Could you check a few things on this model? Use its own coordinates, in mm. A direction names the side the tool comes from. Coordinates: 2 decimals unless noted, no trailing zeros. Order: outer loops, then holes, each group sorted by start corner. A loop starts at its lowest first (then second) coordinate and runs counter-clockwise, first axis right, second up.
```python
from build123d import *

# Parameters (mm, degrees)
SKETCH1_R                  = 25.4
BOSS_EXTRUDE1_DEPTH        = 25.4
CUT_EXTRUDE1_START         = -12.7
SKETCH2_R                  = 25.4
SKETCH2_R_2                = 15.875
CUT_EXTRUDE1_DEPTH         = 12.7
F_3_4_0_7500_DOWEL_HOLE1_D = 19.05
F_3_0MM_DOWEL_HOLE1_D      = 3
CRVPATTERN1_OUTLINE_R      = 1.5
CRVPATTERN1_DEPTH          = 12.7


# Read off the part's stored shape, not the designer's step: CrvPattern1
with BuildPart() as part:
    # Sketch1 → Boss-Extrude1 (new body)
    with BuildSketch(Plane.XY):
        Circle(SKETCH1_R)
    extrude(amount=BOSS_EXTRUDE1_DEPTH)

    # Sketch2 → Cut-Extrude1 (cut)
    with BuildSketch(Plane.XY.offset(25.4).offset(CUT_EXTRUDE1_START)):
        Circle(SKETCH2_R)
        Circle(SKETCH2_R_2, mode=Mode.SUBTRACT)
    extrude(amount=CUT_EXTRUDE1_DEPTH, mode=Mode.SUBTRACT)

    # 3/4 (0.7500) Dowel Hole1 (through all)
    with Locations(Plane.XY.offset(25.4)):
        with Locations((0, 0)):
            Hole(F_3_4_0_7500_DOWEL_HOLE1_D / 2)

    # Ø3.0mm Dowel Hole1 (through all)
    with Locations(Plane(origin=(-0.272270363, 20.318175825, 12.7), x_dir=(1, 0, 0), z_dir=(0, 0, 1))):
        with Locations((0, 0)):
            Hole(F_3_0MM_DOWEL_HOLE1_D / 2)

    # CrvPattern1 outline → CrvPattern1 (cut)
    with BuildSketch(Plane.XY):
        with Locations((-20.318175825, -0.272270363)):
            Circle(CRVPATTERN1_OUTLINE_R)
        with Locations((0.272270363, -20.318175825)):
            Circle(CRVPATTERN1_OUTLINE_R)
        with Locations((20.318175825, 0.272270363)):
            Circle(CRVPATTERN1_OUTLINE_R)
    extrude(amount=CRVPATTERN1_DEPTH, mode=Mode.SUBTRACT)


solid = part.part
```
Item 1: Suppose I cut it at A-A (x = 0). List the corners of the cut face in (y, z) for me (3 decimals), and give its area (3 significant figures).
Item 2: I need wall thicknesses on line 1 (Z direction, x = 14.5, y = -8.5); line 2 (Y direction, x = -4.5, z = 12); line 3 (Y direction, x = -8, z = 15.25). Which ranges of each line are inside material? Lowest first, please.
Item 3: Which directions (+Z, -Z, +X, -X, +Y, -Y) give clear straight access to the entire face, cutting with the end or side of a thin tool? Please do faces 4 (the face through (-1.08, 21.58, 6.26)), 5 (the face through (11, 12, 12.7)).
Item 4: Thinking about a two-plate mould opening in X: for faces 1 (the face through (-3.441, -15.497, 18.961)), 2 (the face through (7, -7, 25.4)), 3 (the face through (18.82, 0.34, 6.26)), which applies, +X half, -X half, draft (parallel to the pull), parting line (faces both ways), or undercut?
Item 5: Suppose I cut it at C-C (z = 16.5). List the corners of the cut face in (x, y) for me (3 decimals).
Item 6: Suppose I cut it at D-D (x = 14). List the corners of the cut face in (y, z) for me.
Item 7: For pin 1 Ø5 at (x, y) = (19.5, -11) entering from +Z; pin 2 Ø1 at (x, z) = (7.5, 5.5) entering from +Y; pin 3 Ø2.5 at (x, y) = (-0.27, 20.32) entering from +Z; pin 4 Ø12 at (y, z) = (-5, 17.5) entering from +X, each with a flat end and sliding along its axis, tell me the tip position at first contact or that it passes through.
Item 8: Suppose I cut it at B-B (y = -19.5). List the corners of the cut face in (x, z) for me, and give its area (3 significant figures).
Geometry results:
1. outline: (-25.4, 0) - (-21.793, 0) - (-21.793, 12.7) - (-25.4, 12.7) - close; (-18.843, 0) - (-9.525, 0) - (-9.525, 25.4) - (-15.875, 25.4) - (-15.875, 12.7) - (-18.843, 12.7) - close; (9.525, 0) - (18.843, 0) - (18.843, 12.7) - (15.875, 12.7) - (15.875, 25.4) - (9.525, 25.4) - close; (21.793, 0) - (25.4, 0) - (25.4, 12.7) - (21.793, 12.7) - close
1. area: 490 mm2
2. line 1: z = 0 to 12.7
2. line 2: y = -25 to -8.39, 8.39 to 25
2. line 3: y = -13.71 to -5.17, 5.17 to 13.71
3. face 4: +Z, -Z
3. face 5: +Z
4. face 1: parting line
4. face 2: draft
4. face 3: undercut
5. outline: circle Ø31.75 at (0, 0); hole circle Ø19.05 at (0, 0)
6. outline: (-21.19, 0) - (21.19, 0) - (21.19, 12.7) - (7.48, 12.7) - (7.48, 25.4) - (-7.48, 25.4) - (-7.48, 12.7) - (-21.19, 12.7) - close
7. pin 1: stops at z = 12.7
7. pin 2: stops at y = 24.42
7. pin 3: passes through
7. pin 4: stops at x = 25.36
8. outline: (-16.28, 0) - (-0.98, 0) - (-0.98, 12.7) - (-16.28, 12.7) - close; (1.53, 0) - (16.28, 0) - (16.28, 12.7) - (1.53, 12.7) - close
8. area: 381 mm2
